Here's the drawing with two shaded views (mm, measured from the low corner). I have some questions. A direction names the side the tool comes from. Give positions to 0.01 mm unless a question says otherwise; leave off trailing zeros. Loops run counter-clockwise (first coordinate to the right, second up) from the corner with the lowest first, then second, coordinate; pieces in that order, holes last. Notation, with made-up numbers: M -33.75,-26.75 L 10.25,-26.75 A17 ccw 10.25,6.25 Z; hole C 57,55 d8. An arc over 180 degrees is marked long. Write item = value, one per line. Start each with the question number.
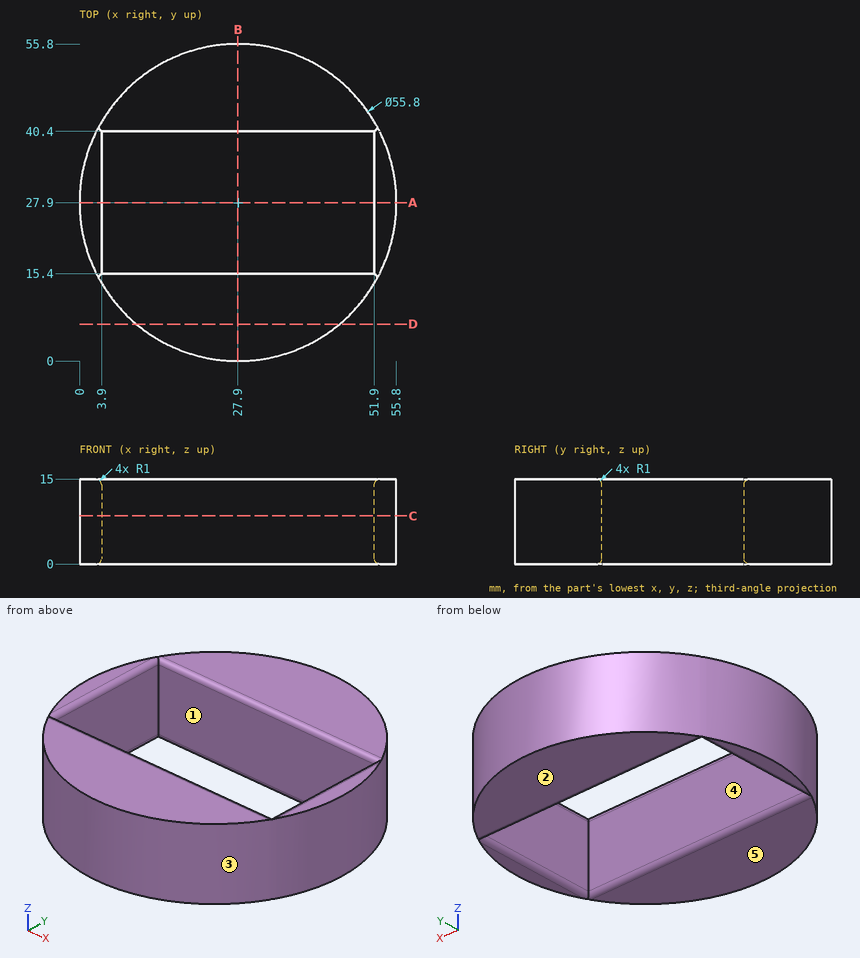
Q1. If I drill on line 1 along Y through (x, z) = (19.5, 12.75); line 2 along Y through (x, z) = (15, 13.25); line 3 along X through (y, z) = (40, 3.5), over which ranges is the centre line in solid material (lowest first)?
Q2. If we section it at C-C, the plane z = 8.5: List the corners of the cut face in (x, y) for me.
Q3. We'd pull the mould along Y, two halves only. Please class the marked faces 1, 2 and 3: pulls with the +Y half, pulls with the -Y half, needs draft (parallel to the pull), parting line crosses it, or undercut.
Q4. If we section it at D-D, the plane y = 6.5: List the corners of the cut face in (x, z) for me, then the cut area to 3 significant figures.
Q5. Will these pins go through, and if not, where does the flat tip stop? pin 1 (1.5 mm diameter, centred on x = 46, z = 2, fed in from -Y); pin 2 (1.5 mm diameter, centred on y = 31.5, z = 13, fed in from +X); pin 3 (6 mm diameter, centred on y = 47, z = 7.5, fed in from +X).
Q6. On a 3-axis mill with a long thin cutter (end or side, diameter ignored), from which of +Z, -Z, +X, -X, +Y, -Y can I reach the whole of each face in a straight line? I mean the marked faces 4 and 5. Say none if no direction works.
Q7. If we section it at B-B, the plane x = 27.9: List the corners of the cut face in (y, z) for me.
Q8. If we section it at A-A, the plane y = 27.9: List the corners of the cut face in (x, z) for me, then the cut area to 3 significant figures.
Resolved:
q1.line_1 = 1.29 to 15.4, 40.4 to 54.51
q1.line_2 = 3.16 to 15.4, 40.4 to 52.64
q1.line_3 = 2.76 to 3.9, 51.9 to 53.04
q2.outline = C 27.9,27.9 d55.8; hole M 3.9,15.4 L 51.9,15.4 L 51.9,40.4 L 3.9,40.4 Z
q3.face_1 = undercut
q3.face_2 = needs draft
q3.face_3 = parting line crosses it
q4.outline = M 10,0 L 45.8,0 L 45.8,15 L 10,15 Z
q4.area = 537 mm²
q5.pin_1 = 6.05
q5.pin_2 = 55.65
q5.pin_3 = 50.69
q6.face_4 = +Z, -Z
q6.face_5 = -Z, +X, -X, +Y, -Y
q7.outline = M 0,0 L 14.4,0 A1 ccw 15.4,1 L 15.4,14 A1 ccw 14.4,15 L 0,15 Z; M 40.4,1 A1 ccw 41.4,0 L 55.8,0 L 55.8,15 L 41.4,15 A1 ccw 40.4,14 Z
q8.outline = M 0,0 L 2.9,0 A1 ccw 3.9,1 L 3.9,14 A1 ccw 2.9,15 L 0,15 Z; M 51.9,1 A1 ccw 52.9,0 L 55.8,0 L 55.8,15 L 52.9,15 A1 ccw 51.9,14 Z
q8.area = 116 mm²
